from build123d import *

# Parameters (mm, degrees)
SKETCH1_R   = 6.35
SKETCH1_R_2 = 5.5372


with BuildPart() as part:
    # Sweep1: sweep along a path in Sketch2
    with BuildLine(Plane(origin=(0, 0, 0), x_dir=(0, 0, -1), z_dir=(1, 0, 0))) as sweep1_path:
        Line((0, 0), (152.4, 0))
        ThreePointArc((152.4, 0), (188.321024484, -14.878975516), (203.2, -50.8))
        Line((203.2, -50.8), (203.2, -340.36))
    # Sketch1 → Sweep1 (sweep)
    with BuildSketch(Plane.XY):
        Circle(SKETCH1_R)
        Circle(SKETCH1_R_2, mode=Mode.SUBTRACT)
    sweep(path=sweep1_path.line)

    # Sketch3 → Revolve1 (revolve)
    with BuildSketch(Plane(origin=(0, 0, 0), x_dir=(0, 0, -1), z_dir=(1, 0, 0))):
        Polygon((0, 5.5372), (-1.122532015, 6.659732015), (-1.122532015, 7.472532015), (0, 6.35), align=None)
    revolve(axis=Axis((0, 0, -10.129320082), (0, 0, 1)))

    # Sketch4 → Revolve2 (revolve)
    with BuildSketch(Plane(origin=(0, 0, 0), x_dir=(0, 0, -1), z_dir=(1, 0, 0)), mode=Mode.PRIVATE) as revolve2_sk:
        Polygon((196.85, -340.36), (188.107467985, -349.102532015), (188.920267985, -349.102532015), (197.6628, -340.36), align=None)
    revolve(revolve2_sk.sketch.rotate(Axis((0, -309.261339279, -203.2), (0, -1, 0)), 180), axis=Axis((0, -309.261339279, -203.2), (0, -1, 0)))


solid = part.part
Model file for the job. Use its own axes, mm. A direction names the side the tool comes from. Give positions to 0.01 mm unless a question says otherwise; leave off trailing zeros. Loops run counter-clockwise (first coordinate to the right, second up) from the corner with the lowest first, then second, coordinate; pieces in that order, holes last.
1) Tool access for faces 1 (the cylindrical face through (-4.394, 3.369, -77.267)), 2 (the conical face through (2.07, -340.91, -209.78)), 3 (the flat face through (1, 7, 1.123)): list every direction of +Z, -Z, +X, -X, +Y, -Y with a clear straight run to the whole face (end or side of a thin tool).
2) Saw through at C-C (y = -207). Write the cut outline in (x, z), plus the area to 3 significant figures.
3) Flat gauge pins, fed straight in: pin 1 Ø10 at (x, z) = (3.5, -100.5) entering from +Y; pin 2 Ø9 at (x, z) = (0, -203.2) entering from +Y; pin 3 Ø9 at (x, y) = (0, 0) entering from -Z. Where does each tip first touch, or does it go through?
4) Saw through at A-A (x = 0). Write the cut outline in (y, z), plus the area to 3 significant figures.
5) Pull direction Z, two halves, no side cores. Call faces 4 (the cylindrical face through (-1.38, -197.61, -209.4)), 5 (the flat face through (-13.35, -349.103, -208.72)), 6 (the cylindrical face through (-1.2, -197.607, -208.606)): +Z half, -Z half, draft (parallel to the pull), parting line (faces both ways), or undercut.
6) Wall check: line 1 (Z direction, x = -0.5, y = -104); line 2 (X direction, y = 0, z = -77.5). Give the ranges that are in metal, low to high.
7) Saw through at B-B (z = -23.5). Write the cut outline in (x, y).
Answer block:
1. face 1: +Z
1. face 2: none
1. face 3: +Z, +X, -X, +Y, -Y
2. outline: circle Ø12.7 at (0, -203.2); hole circle Ø11.07 at (0, -203.2)
2. area: 30.4 mm2
3. pin 1: stops at y = 6.35
3. pin 2: stops at y = -17.3
3. pin 3: stops at z = -185.9
4. outline: (-349.1, -218.29) - (-340.36, -209.55) - (-50.8, -209.55) arc R57.15 ccw to (6.35, -152.4) - (6.35, 0) - (7.47, 1.12) - (6.66, 1.12) - (5.54, 0) - (5.54, -152.4) arc R56.34 cw to (-50.8, -208.74) - (-340.36, -208.74) - (-349.1, -217.48) - close; (-349.1, -188.92) - (-340.36, -197.66) - (-50.8, -197.66) arc R45.26 ccw to (-5.54, -152.4) - (-5.54, 0) - (-6.66, 1.12) - (-7.47, 1.12) - (-6.35, 0) - (-6.35, -152.4) arc R44.45 cw to (-50.8, -196.85) - (-340.36, -196.85) - (-349.1, -188.11) - close
4. area: 864 mm2
5. face 4: parting line
5. face 5: draft
5. face 6: undercut
6. line 1: z = -209.53 to -208.71, -197.69 to -196.87
6. line 2: x = -6.35 to -5.54, 5.54 to 6.35
7. outline: circle Ø12.7 at (0, 0); hole circle Ø11.07 at (0, 0)
